Design review of the part shown in the three views and the two pictorial views. Dimensions are in mm from the part's minimum x, y and z. Coordinates: 2 decimals unless noted, no trailing zeros. Loops run counter-clockwise (first coordinate to the right, second up) from the corner with the lowest first, then second, coordinate; pieces in that order, holes last. Notation, with made-up numbers: M 7,59 L 20,59 A27 ccw 20,87 Z; hole C -15.5,-20 d10. An arc over 180 degrees is marked long. Use CSV: the item, a comma, the result in double quotes. Start each with the question number.
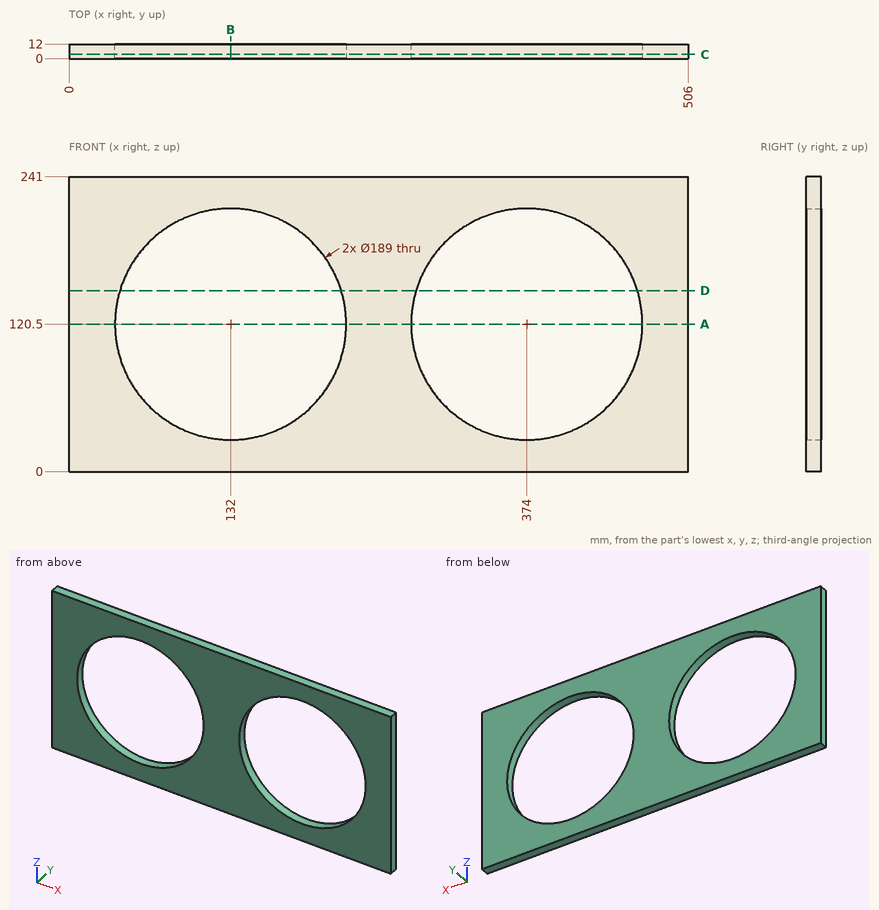
1. Add section A-A (z = 120.5). Write out the cut boundary in (x, y), plus the area to 3 significant figures.
2. Add section C-C (y = 3.5). Write out the cut boundary in (x, z), plus the area to 3 significant figures.
3. To check wall thickness, follow line 1 along X through (y, z) = (8, 144); line 2 along X through (y, z) = (4.5, 197.5); line 3 along Z through (x, y) = (132, 7). State the ranges of each line that lie inside material, in increasing order.
4. Add section D-D (z = 148). Write out the cut boundary in (x, y), plus the area to 3 significant figures.
5. Insertion check: pin 1 Ø12 at (x, z) = (214.5, 130) entering from -Y. The pin has a flat end and moves straight along its axis. Give the tip position at first contact, or say it passes through.
6. Add section B-B (x = 132). Write out the cut boundary in (y, z), plus the area to 3 significant figures.
Solved:
1,outline,"M 0,0 L 37.5,0 L 37.5,12 L 0,12 Z; M 226.5,0 L 279.5,0 L 279.5,12 L 226.5,12 Z; M 468.5,0 L 506,0 L 506,12 L 468.5,12 Z"
1,area,"1,540 mm^2"
2,outline,"M 0,0 L 506,0 L 506,241 L 0,241 Z; hole C 132,120.5 d189; hole C 374,120.5 d189"
2,area,"65,800 mm^2"
3,line 1,"x = 0 to 40.47, 223.53 to 282.47, 465.53 to 506"
3,line 2,"x = 0 to 77.22, 186.78 to 319.22, 428.78 to 506"
3,line 3,"z = 0 to 26, 215 to 241"
4,outline,"M 0,0 L 41.59,0 L 41.59,12 L 0,12 Z; M 222.41,0 L 283.59,0 L 283.59,12 L 222.41,12 Z; M 464.41,0 L 506,0 L 506,12 L 464.41,12 Z"
4,area,"1,730 mm^2"
5,pin 1,"passes through"
6,outline,"M 0,0 L 12,0 L 12,26 L 0,26 Z; M 0,215 L 12,215 L 12,241 L 0,241 Z"
6,area,"624 mm^2"
